Autodesk Inventor part; units mm, degrees
ref_plane "YZ Plane" through (0, 0, 0) normal (1, 0, 0) x (0, 1, 0)
ref_plane "XZ Plane" through (0, 0, 0) normal (0, 1, 0) x (-1, 0, 0)
ref_plane "XY Plane" through (0, 0, 0) normal (0, 0, 1) x (1, 0, 0)
sketch "Sketch1" plane through (0, 0, 0) normal (0, 1, 0) x (-1, 0, 0)
  line L0 (0, 0) -> (-5.08, 0)
  line L1 (-5.08, 0) -> (-5.08, -15.24)
  line L2 (-5.08, -15.24) -> (0, -15.24)
  line L3 (0, -15.24) -> (0, 0)
  line L4 (-5.08, -7.62) -> (-5.08, -5.08)
  line L5 (-5.08, -5.08) -> (-8.89, -5.08)
  line L6 (-8.89, -5.08) -> (-8.89, -2.54)
  line L7 (-8.89, -5.08) -> (-11.43, -5.08)
  line L8 (-11.43, -5.08) -> (-11.43, -10.16)
  line L9 (-11.43, -10.16) -> (-5.08, -10.16)
  line L10 (-8.89, -10.16) -> (-8.89, -12.7)
  line L11 (-8.89, -12.7) -> (-11.43, -10.16)
  line L12 (-8.89, -2.54) -> (-11.43, -5.08)
  dimension "d0" = 5.08
  dimension "d1" = 15.24
  dimension "d2" = 2.54
  dimension "d3" = 3.81
  dimension "d4" = 2.54
  dimension "d5" = 2.54
  dimension "d6" = 5.08
  dimension "d7" = 2.54
extrude "Extrusion1" add sketch "Sketch1" along normal blind 38.1
sketch "Sketch2" plane through (0, 0, -15.24) normal (-1, 0, 0) x (0, 0, 1)
  line L0 (10.16, 0) -> (5.08, 0)
  line L1 (7.62, 0) -> (7.62, 7.62)
  line L2 (10.16, 38.1) -> (5.08, 38.1)
  line L3 (7.62, 38.1) -> (7.62, 30.48)
  point P0 (15.24, 0)
  dimension "d10" = 7.62
  dimension "d11" = 7.62
hole "Hole1" at (0, 7.62, -7.62) at (0, 30.48, -7.62) direction (1, 0, 0) diameter 5.08 end through all counterbore diameter 10.16 counterbore depth 3.81
sketch "Sketch3" plane through (0, 0, -15.24) normal (-1, 0, 0) x (0, 0, 1)
  circle A0 centre (7.62, 7.62) radius 5.08
  circle A1 centre (7.62, 30.48) radius 5.08
  line L0 (0, 0) -> (0, 38.1)
  line L1 (15.24, 0) -> (15.24, 38.1)
  line L2 (0, 12.7) -> (15.24, 12.7)
  line L3 (15.24, 12.7) -> (15.24, 25.4)
  line L4 (15.24, 25.4) -> (0, 25.4)
  line L5 (0, 25.4) -> (0, 12.7)
  dimension "d19" = 12.7
  dimension "d20" = 12.7
extrude "Extrusion2" add sketch "Sketch3" along normal blind 5.08 contours L2 L0 L4 L1
sketch "Sketch4" plane through (5.08, 0, -15.24) normal (0, 0, -1) x (-1, 0, 0)
  line L0 (10.16, 12.7) -> (10.16, 25.4)
  line L1 (10.16, 12.7) -> (8.89, 12.7)
  line L2 (8.89, 12.7) -> (8.89, 13.97)
  line L3 (8.89, 13.97) -> (10.16, 13.97)
  line L4 (10.16, 13.97) -> (10.16, 12.7)
  line L5 (8.89, 13.97) -> (3.81, 13.97)
  line L6 (3.81, 13.97) -> (3.81, 24.13)
  line L7 (3.81, 24.13) -> (8.89, 24.13)
  line L8 (8.89, 24.13) -> (8.89, 13.97)
  point P0 (5.08, 0)
  dimension "d23" = 1.27
  dimension "d24" = 1.27
  dimension "d25" = 5.08
  dimension "d26" = 10.16
extrude "Extrusion3" cut sketch "Sketch4" against normal blind 15.24 contours L5 L6 L7 L8
properties part number "Mount Female"
Geometry: final body of the model. Coordinates: model frame, mm. A direction names the side the tool comes from. Give positions to 0.01 mm unless a question says otherwise; leave off trailing zeros. Write each loop counter-clockwise with the first axis right and the second up, starting at its lowest first coordinate (ties: lowest second). Pieces come first, ordered by that corner, then holes. Notation, with made-up numbers: (-23.75, 6.25) -> (-3.75, 6.25) arc R22 cw to (-3.75, 12.25) -> close; hole circle Ø10 at (56.25, -16.75). An arc over 180 degrees is marked (long way). Answer in a Markdown table with one row per item.
(1) Section query D-D on x = -3.25. Return loops of the section in (y, z), then the cut area to 3 significant figures.
Answers below:
| item | result |
|---|---|
| outline | (12.7, -15.24) -> (13.97, -15.24) -> (13.97, 0) -> (12.7, 0) -> close; (24.13, -15.24) -> (25.4, -15.24) -> (25.4, 0) -> (24.13, 0) -> close |
| area | 38.7 mm^2 |
(2) Ray query, line 1 along Y through (x, z) = (10.25, -7.62); line 2 along Y through (x, z) = (2.8, -7.62); line 3 along X through (y, z) = (21, -11.5). Return the intervals inside material, ascending. Write a range as [from, to].
Answers below:
| item | result |
|---|---|
| line 1 | [0, 5.08], [10.16, 27.94], [33.02, 38.1] |
| line 2 | [0, 2.54], [12.7, 25.4], [35.56, 38.1] |
| line 3 | [-5.08, -3.81], [1.27, 5.08], [8.89, 10.09] |
(3) Section query A-A on y = 22.5. Return loops of the section in (x, z).
Answers below:
| item | result |
|---|---|
| outline | (-5.08, -15.24) -> (-3.81, -15.24) -> (-3.81, 0) -> (-5.08, 0) -> close; (1.27, -15.24) -> (5.08, -15.24) -> (5.08, -10.16) -> (8.89, -10.16) -> (8.89, -12.7) -> (11.43, -10.16) -> (11.43, -5.08) -> (8.89, -2.54) -> (8.89, -5.08) -> (5.08, -5.08) -> (5.08, 0) -> (1.27, 0) -> close |
(4) Draft query along Z for faces 1 (the cylindrical face through (1.93, 35.44, -8.72)), 2 (the flat face through (1.27, 19, -8)), 3 (the flat face through (10.14, 18.78, -3.79)), 4 (the cylindrical face through (1.93, 10.71, -11.65)). Return one class per face: +Z half, -Z half, draft (parallel to the pull), parting line (faces both ways), or undercut.
Answers below:
| item | result |
|---|---|
| face 1 | undercut |
| face 2 | draft |
| face 3 | +Z half |
| face 4 | undercut |
(5) Pin query (flat end, axial travel): pin 1 (1.5 mm diameter, centred on x = -1.5, z = -9.5, fed in from +Y); pin 2 (2 mm diameter, centred on x = 3, z = -2, fed in from -Y); pin 3 (6 mm diameter, centred on y = 7.62, z = -7.62, fed in from -X); pin 4 (3 mm diameter, centred on x = 7, y = 5, fed in from +Z). Return the tip coordinate at first contact, or that it passes through.
Answers below:
| item | result |
|---|---|
| pin 1 | y = 25.4 |
| pin 2 | y = 0 |
| pin 3 | x = 3.81 |
| pin 4 | z = -5.08 |
(6) Set-up query: faces 5 (the flat face through (3.81, 32, -10)), 6 (the flat face through (-3, 12.7, -8)), 7 (the flat face through (0, 36, -8)). Return all of +Z, -Z, +X, -X, +Y, -Y with unobstructed straight access to the full face (end or side cutting, diameter ignored); none if empty.
Answers below:
| item | result |
|---|---|
| face 5 | -X |
| face 6 | +Z, -Z, -X, -Y |
| face 7 | +Z, -Z, -X, +Y |
(7) Section query C-C on z = -3.75. Return loops of the section in (x, y).
Answers below:
| item | result |
|---|---|
| outline | (-5.08, 12.7) -> (0, 12.7) -> (0, 10.91) -> (3.81, 10.91) -> (3.81, 4.33) -> (0, 4.33) -> (0, 0) -> (5.08, 0) -> (5.08, 38.1) -> (0, 38.1) -> (0, 33.77) -> (3.81, 33.77) -> (3.81, 27.19) -> (0, 27.19) -> (0, 25.4) -> (-5.08, 25.4) -> close; (8.89, 0) -> (10.1, 0) -> (10.1, 38.1) -> (8.89, 38.1) -> close; hole (-3.81, 13.97) -> (1.27, 13.97) -> (1.27, 24.13) -> (-3.81, 24.13) -> close |
